Autodesk Inventor part; units mm, degrees
ref_plane "Work Plane1" through (57.5, 10, 0) normal (1, 0, 0) x (0, 1, 0)
ref_plane "XZ Plane" through (0, 0, 0) normal (0, 1, 0) x (-1, 0, 0)
ref_plane "XY Plane" through (0, 0, 0) normal (0, 0, 1) x (1, 0, 0)
sketch "Sketch1" plane through (0, 0, 0) normal (0, 1, 0) x (-1, 0, 0)
  circle A0 centre (0, 0) radius 4
  circle A1 centre (0, 0) radius 12
  dimension "d0" = 8
  dimension "d1" = 24
extrude "Extrusion1" add sketch "Sketch1" along normal blind 10
sketch "Sketch2" plane through (0, 10, 0) normal (0, 1, 0) x (1, 0, 0)
  circle A0 centre (0, 0) radius 12
  line L0 (1.08, 11.9513) -> (50.675, 7.4696)
  circle A1 centre (50, 0) radius 7.5
  line L1 (50.675, -7.4696) -> (1.08, -11.9513)
  circle A2 centre (50, 0) radius 2.7
  circle A3 centre (0, 0) radius 12
  point P0 (3.9985, -10.2475)
  point P1 (1.1339, 10.9414)
  dimension "d4" = 50
  dimension "d5" = 15
  dimension "d6" = 5.4
extrude "Extrusion2" add sketch "Sketch2" against normal up to surface (10 mm away) contours A0 L0 A1 L1 | A1
sketch "Sketch3" plane through (0, 10, 0) normal (0, 1, 0) x (1, 0, 0)
  circle A0 centre (0, 0) radius 7.1
  line L0 (8.1984, 0) -> (4.0992, -7.1)
  line L1 (4.0992, -7.1) -> (-4.0992, -7.1)
  line L2 (-4.0992, -7.1) -> (-8.1984, 0)
  line L3 (-8.1984, 0) -> (-4.0992, 7.1)
  line L4 (-4.0992, 7.1) -> (4.0992, 7.1)
  line L5 (4.0992, 7.1) -> (8.1984, 0)
  dimension "d9" = 14.2
extrude "Extrusion3" cut sketch "Sketch3" against normal blind 10
ref_plane "Work Plane1" through (57.5, 10, 0) normal (1, 0, 0) x (0, 1, 0)
sketch "Sketch4" plane through (57.5, 10, 0) normal (1, 0, 0) x (0, 1, 0)
  line L0 (-2.9, -4.1) -> (-7.1, -4.1)
  line L1 (-7.1, -4.1) -> (-7.1, 4.1)
  line L2 (-7.1, 4.1) -> (-2.9, 4.1)
  line L3 (-2.9, 4.1) -> (-2.9, -4.1)
  line L4 (0, 0) -> (-10, 0)
  line L5 (-2.9, -4.1) -> (-7.1, 4.1) construction
  line L6 (-7.1, -4.1) -> (-2.9, 4.1) construction
  point P0 (-5, 0)
  dimension "d12" = 4.2
  dimension "d13" = 8.2
extrude "Extrusion4" cut sketch "Sketch4" against normal blind 12.5
chamfer "Chamfer1" distance 3 angle 30 2 edges at (45, 5, -4.1) (45, 5, 4.1) measured on face at (45, 4.3, -1.3667)
fillet "Fillet1" radius 1 8 edges at (-12, 0, 0) (25.8775, 0, -9.7104) (57.5, 0, 0) (25.8775, 0, 9.7104) (57.5, 10, 0) (25.8775, 10, -9.7104) (-12, 10, 0) (25.8775, 10, 9.7104)
properties part number "Crank"
Geometry: final body of the model. Coordinates: model frame, mm. A direction names the side the tool comes from. Round coordinates to 2 decimals unless told otherwise and drop trailing zeros. Order: outer loops, then holes, each group sorted by start corner. A loop starts at its lowest first (then second) coordinate and runs counter-clockwise, first axis right, second up. Notation, with made-up numbers: M 62.5,3.5 L 93.5,3.5 A24 cw 93.5,29.5 Z; hole C 15,36 d6. An arc over 180 degrees is marked long. Use one line per item in the form item = value. Start each with the question number.
Q1. Mould query, pull axis X, two halves, no side actions, for faces 4 (the face through (0, 5, 7.1)), 5 (the face through (0, 5, -7.1)), 6 (the face through (53, 7.1, 0)), 7 (the face through (57.5, 2.39, 0.16)). Classes: +X half, -X half, draft (parallel to the pull), parting line (faces both ways), or undercut.
Q2. Material intervals for line 1 (X direction, y = 8, z = 0); line 2 (X direction, y = 1, z = -0.25); line 3 (Z direction, x = 50, y = 2.25), sorted ascending. Write a range as [from, to].
Q3. Cut plane A-A (y = 5.75). Return loops of the section in (x, z) (3 decimals).
Q4. Access query for faces 1 (the face through (45.878, 4.971, -2.621)), 2 (the face through (25.53, 5.06, -9.74)), 3 (the face through (-6.12, 5.07, 3.6)). Directions: +Z, -Z, +X, -X, +Y, -Y. A direction counts if a zero-diameter tool reaches every point of the face in a straight line with its end or side. Return the directions, or none.
Q5. Pin query (flat end, axial travel): pin 1 Ø5 at (y, z) = (2.5, -6.5) entering from +X; pin 2 Ø4 at (x, y) = (18.5, 3.5) entering from -Z; pin 3 Ø3 at (x, y) = (43.5, 8) entering from -Z. Return the tip coordinate at first contact, or that it passes through.
Q6. Cut plane B-B (x = 0). Return loops of the section in (y, z).
Geometry results:
q1.face_4 = undercut
q1.face_5 = undercut
q1.face_6 = draft
q1.face_7 = +X half
q2.line_1 = [-12, -8.2], [8.2, 47.3], [52.7, 57.5]
q2.line_2 = [-12, -8.05], [8.05, 47.31], [52.69, 57.5]
q2.line_3 = [-7.53, -2.7], [2.7, 7.53]
q3.outline = M 1.08,-11.951 L 50.675,-7.47 A7.5 ccw 56.28,-4.1 L 46.732,-4.1 L 45,-1.1 L 45,1.1 L 46.732,4.1 L 56.28,4.1 A7.5 ccw 50.675,7.47 L 1.08,11.951 A12 ccw long Z; hole M -8.198,0 L -4.099,-7.1 L 4.099,-7.1 L 8.198,0 L 4.099,7.1 L -4.099,7.1 Z
q4.face_1 = +X
q4.face_2 = -Z, +X, +Y, -Y
q4.face_3 = +Y, -Y
q5.pin_1 = 56.34
q5.pin_2 = -10.56
q5.pin_3 = -8.25
q6.outline = M 0,-11 A1 ccw 1,-12 L 9,-12 A1 ccw 10,-11 L 10,-7.1 L 0,-7.1 Z; M 0,7.1 L 10,7.1 L 10,11 A1 ccw 9,12 L 1,12 A1 ccw 0,11 Z
